Build history of the part. All positions in model axes, mm. Face numbers are marked on the shaded views. A direction names the side the tool comes from. Round coordinates to 2 decimals unless told otherwise and drop trailing zeros. Write each loop counter-clockwise with the first axis right and the second up, starting at its lowest first coordinate (ties: lowest second). Pieces come first, ordered by that corner, then holes. Notation, with made-up numbers: M -28.5,-30.5 L 28.5,-30.5 A19 cw 28.5,5.5 Z; hole C -1,81.5 d9. An arc over 180 degrees is marked long. Write item = value, one per line.
Autodesk Inventor part; units mm, degrees
ref_plane "YZ Plane" through (0, 0, 0) normal (1, 0, 0) x (0, 1, 0)
ref_plane "XZ Plane" through (0, 0, 0) normal (0, 1, 0) x (-1, 0, 0)
ref_plane "XY Plane" through (0, 0, 0) normal (0, 0, 1) x (1, 0, 0)
sketch "Sketch2" plane through (0, 0, 0) normal (0, 1, 0) x (-1, 0, 0)
  line L0 (10.6557, -7.541) -> (-39.3443, -7.541)
  line L1 (-39.3443, -7.541) -> (-39.3443, 12.459)
  line L2 (-39.3443, 12.459) -> (10.6557, 12.459)
  line L3 (10.6557, 12.459) -> (10.6557, -7.541)
  point P0 (0, 0)
  dimension "d10" = 20
  dimension "d11" = 50
extrude "Extrusion3" add sketch "Sketch2" along normal blind 10
sketch "Sketch3" plane through (0, 10, 0) normal (0, 1, 0) x (1, 0, 0)
  line L0 (39.3443, 7.541) -> (-10.6557, 7.541)
  line L1 (-10.6557, 7.541) -> (-10.6557, -12.459)
  line L2 (-10.6557, -12.459) -> (39.3443, -12.459)
  line L3 (39.3443, -12.459) -> (39.3443, 7.541)
  line L4 (-1.6557, -10.959) -> (-1.6557, 7.041)
  line L5 (-1.6557, 7.041) -> (30.3443, 7.041)
  line L6 (30.3443, 7.041) -> (30.3443, -10.959)
  line L7 (30.3443, -10.959) -> (25.3443, -10.959)
  line L8 (25.3443, -10.959) -> (25.3443, 2.041)
  line L9 (25.3443, 2.041) -> (3.3443, 2.041)
  line L10 (3.3443, 2.041) -> (3.3443, -10.959)
  line L11 (3.3443, -10.959) -> (-1.6557, -10.959)
  line L12 (-1.6557, 7.041) -> (-10.6557, 7.041) construction
  line L13 (30.3443, 7.041) -> (39.3443, 7.041) construction
  line L14 (-1.6557, 7.041) -> (-1.6557, 7.541) construction
  point P0 (0, 0)
  dimension "d14" = 22
  dimension "d15" = 5
  dimension "d16" = 5
  dimension "d17" = 0.5
  dimension "d18" = 13
extrude "Extrusion4" add sketch "Sketch3" along normal blind 55 contours L4 L5 L6 L7 L8 L9 L10 L11
sketch "Sketch4" plane through (30.3443, 10, -7.041) normal (0, 0, -1) x (-1, 0, 0)
  circle A0 centre (16, 34.875) radius 2.125
  line L0 (16, 34.875) -> (0, 34.875) construction
  line L1 (0, 0) -> (0, 55)
  line L2 (16, 34.875) -> (32, 34.875) construction
  line L3 (32, 0) -> (32, 55)
  line L4 (0, 55) -> (32, 55)
  line L5 (-9, 0) -> (41, 0)
  point P0 (30.3443, -10)
  point P1 (28, 0)
  dimension "d21" = 4.25
  dimension "d32" = 34.875
extrude "Extrusion5" cut sketch "Sketch4" against normal up to next contours A0
sketch "Sketch5" plane through (0, 10, 0) normal (0, 1, 0) x (1, 0, 0)
  circle A0 centre (-5.6557, -2.459) radius 2.125
  circle A1 centre (34.3443, -2.459) radius 2.125
  line L0 (-5.6557, -2.459) -> (-10.6557, -2.459) construction
  line L1 (34.3443, -2.459) -> (39.3443, -2.459) construction
  line L2 (39.3443, -12.459) -> (39.3443, 7.541)
  line L3 (39.3443, 7.541) -> (-10.6557, 7.541)
  line L4 (-10.6557, 7.541) -> (-10.6557, -12.459)
  point P0 (0, 0)
  dimension "d26" = 4.25
  dimension "d27" = 10
  dimension "d28" = 5
extrude "Extrusion6" cut sketch "Sketch5" against normal up to next
sketch "Sketch6" plane through (30.3443, 10, 10.959) normal (1, 0, 0) x (0, 0, -1)
  circle A0 centre (2.8, 31) radius 1.625
  circle A1 centre (2.8, 50) radius 1.625
  line L0 (18, 0) -> (0, 0)
  line L1 (0, 0) -> (0, 55)
  line L2 (2.8, 50) -> (2.8, 31) construction
  point P0 (10.959, -10)
  dimension "d33" = 3.25
  dimension "d34" = 3.25
  dimension "d35" = 19
  dimension "d36" = 31
  dimension "d37" = 2.8
extrude "Extrusion7" cut sketch "Sketch6" against normal up to surface (5 mm away)
sketch "Sketch7" plane through (25.3443, 10, -2.041) normal (-1, 0, 0) x (0, 0, 1)
  line L0 (0, 55) -> (13, 55)
  line L1 (7, 55) -> (7, 25)
  line L2 (7, 25) -> (13, 25)
  line L3 (13, 0) -> (13, 55)
  line L4 (13, 25) -> (13, 55)
  line L5 (7, 55) -> (13, 55)
  point P0 (2.041, -10)
  dimension "d40" = 6
  dimension "d41" = 30
extrude "Extrusion8" cut sketch "Sketch7" against normal blind 2
properties part number "XPulleySupportBase" material "ABS Plastic"
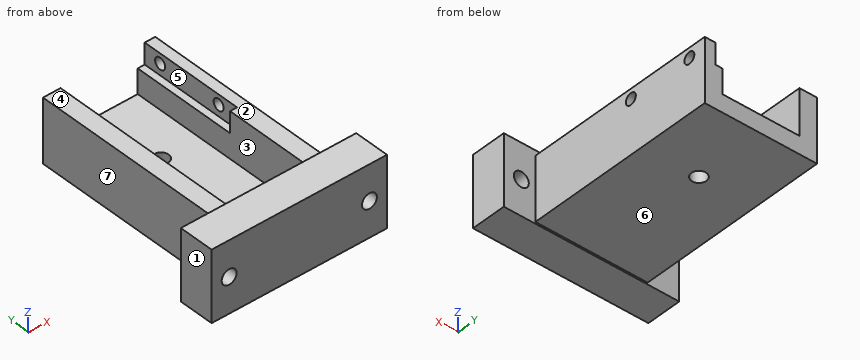
1. Band-saw the part on C-C (y = 23). List the corners of the cut face in (x, z), plus the area to 3 significant figures.
Responses:
outline = M -1.66,-7.04 L 30.34,-7.04 L 30.34,10.96 L 25.34,10.96 L 25.34,-2.04 L 3.34,-2.04 L 3.34,10.96 L -1.66,10.96 Z
area = 290 mm²
2. Mould opens along X. For the marked faces 1, 2 and 3 say: pulls with the +X half, pulls with the -X half, needs draft (parallel to the pull), parting line crosses it, or undercut.
Responses:
face_1 = pulls with the -X half
face_2 = needs draft
face_3 = undercut
3. Band-saw the part on B-B (x = 28.5). List the corners of the cut face in (y, z) (3 decimals), plus the area to 3 significant figures.
Responses:
outline = M 0,-7.541 L 10,-7.541 L 10,-7.041 L 65,-7.041 L 65,10.959 L 10,10.959 L 10,12.459 L 0,12.459 Z; hole C 41,8.159 d3.25; hole C 60,8.159 d3.25
area = 1,170 mm²
4. Flat gauge pins, fed straight in: pin 1 (5 mm diameter, centred on y = 41, z = 8.159, fed in from -X); pin 2 (4 mm diameter, centred on y = 31.5, z = 5.5, fed in from +X); pin 3 (1 mm diameter, centred on x = 26.5, y = 45, fed in from +Z). Where does each tip first touch, or does it go through?
Responses:
pin_1 = -1.66
pin_2 = 30.34
pin_3 = 4.96
5. Band-saw the part on A-A (y = 60). List the corners of the cut face in (x, z), plus the area to 3 significant figures.
Responses:
outline = M -1.66,-7.04 L 30.34,-7.04 L 30.34,6.53 L 27.34,6.53 L 27.34,4.96 L 25.34,4.96 L 25.34,-2.04 L 3.34,-2.04 L 3.34,10.96 L -1.66,10.96 Z; M 27.34,9.78 L 30.34,9.78 L 30.34,10.96 L 27.34,10.96 Z
area = 268 mm²
6. Band-saw the part on D-D (x = 34.5). List the corners of the cut face in (y, z).
Responses:
outline = M 0,-7.54 L 10,-7.54 L 10,0.34 L 0,0.34 Z; M 0,4.58 L 10,4.58 L 10,12.46 L 0,12.46 Z
7. Probe probe 1 along X at (y, z) = (48, 7.5); probe 2 along X at (y, z) = (40, -0.25); probe 3 along X at (y, z) = (5, 1). List the from-to ranges inside material, lowest first.
Responses:
probe_1 = -1.66 to 3.34, 27.34 to 30.34
probe_2 = -1.66 to 3.34, 25.34 to 30.34
probe_3 = -10.66 to -7.2, -4.11 to 32.8, 35.89 to 39.34
8. Tool access for the marked faces 4, 5, 6 and 7: list every direction of +Z, -Z, +X, -X, +Y, -Y with a clear straight run to the whole face (end or side of a thin tool).
Responses:
face_4 = +Z, +X, -X, +Y
face_5 = +Z, +Y
face_6 = -Z, +X, -X, +Y
face_7 = +Z, -Z, -X, +Y
